```python
from build123d import *

# Parameters (mm, degrees)
BOSS_EXTRUDE1_DEPTH      = 25.5
BOSS_EXTRUDE1_DEPTH_BACK = 25.5
BOSS_EXTRUDE2_DEPTH      = 4
BOSS_EXTRUDE2_DEPTH_BACK = 4
SKETCH3_R                = 10
BOSS_EXTRUDE3_DEPTH      = 12.9
BOSS_EXTRUDE3_DEPTH_BACK = 12.9
SKETCH4_W                = 2.75
SKETCH4_H                = 8
SKETCH5_W                = 2.75
SKETCH5_H                = 8
SKETCH6_W                = 2.75
SKETCH6_H                = 8
SKETCH7_W                = 2.75
SKETCH7_H                = 8


with BuildPart() as part:
    # Sketch1 → Boss-Extrude1 (new body, two sides)
    with BuildSketch(Plane(origin=(0, 0, 0), x_dir=(0, 0, -1), z_dir=(1, 0, 0))) as boss_extrude1_sk:
        with BuildLine():
            Line((-15.5, 6.672), (-15.5, 0))
            Line((-15.5, 0), (15.5, 0))
            Line((15.5, 0), (15.5, 6.672))
            ThreePointArc((15.5, 6.672), (15.111037805, 7.611037805), (14.172, 8))
            Line((14.172, 8), (-14.172, 8))
            ThreePointArc((-14.172, 8), (-15.111037805, 7.611037805), (-15.5, 6.672))
        make_face()
    extrude(amount=BOSS_EXTRUDE1_DEPTH)
    extrude(boss_extrude1_sk.sketch, amount=-BOSS_EXTRUDE1_DEPTH_BACK)

    # Sketch2 → Boss-Extrude2 (add, two sides)
    with BuildSketch(Plane(origin=(0, 0, 0), x_dir=(0, 0, -1), z_dir=(1, 0, 0))) as boss_extrude2_sk:
        with BuildLine():
            Line((-21.283175656, 28.022230556), (-15.5, 6.656))
            ThreePointArc((-15.5, 6.656), (-15.106351514, 7.606351514), (-14.156, 8))
            Line((-14.156, 8), (14.675312578, 8))
            Line((14.675312578, 8), (-2.758705731, 36.074123248))
            ThreePointArc((-2.758705731, 36.074123248), (-2.824497754, 36.091976454), (-2.846947105, 36.027607565))
            ThreePointArc((-2.846947105, 36.027607565), (-8.013665194, 22.828896751), (-21.188967498, 28.055018845))
            ThreePointArc((-21.188967498, 28.055018845), (-21.251347415, 28.082515631), (-21.283175656, 28.022230556))
        make_face()
    extrude(amount=BOSS_EXTRUDE2_DEPTH)
    extrude(boss_extrude2_sk.sketch, amount=-BOSS_EXTRUDE2_DEPTH_BACK)

    # Sketch3 → Boss-Extrude3 (add, two sides)
    with BuildSketch(Plane(origin=(0, 0, 0), x_dir=(0, 0, -1), z_dir=(1, 0, 0))) as boss_extrude3_sk:
        with Locations((-12, 32)):
            Circle(SKETCH3_R)
    extrude(amount=BOSS_EXTRUDE3_DEPTH)
    extrude(boss_extrude3_sk.sketch, amount=-BOSS_EXTRUDE3_DEPTH_BACK)

    # Sketch4 → Cut-Revolve1 (revolve, cut)
    with BuildSketch(Plane.XY.offset(9)):
        with Locations((-20.375, 4)):
            Rectangle(SKETCH4_W, SKETCH4_H)
    revolve(axis=Axis((-19, 8, 9), (0, -1, 0)), mode=Mode.SUBTRACT)

    # Sketch5 → Cut-Revolve2 (revolve, cut)
    with BuildSketch(Plane.XY.offset(9)):
        with Locations((17.625, 4)):
            Rectangle(SKETCH5_W, SKETCH5_H)
    revolve(axis=Axis((19, 8, 9), (0, -1, 0)), mode=Mode.SUBTRACT)

    # Sketch6 → Cut-Revolve3 (revolve, cut)
    with BuildSketch(Plane.XY.offset(-9)):
        with Locations((-20.375, 4)):
            Rectangle(SKETCH6_W, SKETCH6_H)
    revolve(axis=Axis((-19, 8, -9), (0, -1, 0)), mode=Mode.SUBTRACT)

    # Sketch7 → Cut-Revolve4 (revolve, cut)
    with BuildSketch(Plane.XY.offset(-9)):
        with Locations((17.625, 4)):
            Rectangle(SKETCH7_W, SKETCH7_H)
    revolve(axis=Axis((19, 8, -9), (0, -1, 0)), mode=Mode.SUBTRACT)

    # Sketch8 → Cut-Revolve5 (revolve, cut)
    with BuildSketch(Plane.XY.offset(12)):
        Polygon((-12.9, 32), (-12.9, 39.22), (-12.611324865, 38.72), (12.611324865, 38.72), (12.9, 39.22), (12.9, 32), align=None)
    revolve(axis=Axis((12.9, 32, 12), (-1, 0, 0)), mode=Mode.SUBTRACT)

    # Sketch9 → Revolve1 (revolve)
    with BuildSketch(Plane.XY.offset(12)):
        Polygon((-12.9, 37.3), (-12.726794919, 37), (12.726794919, 37), (12.9, 37.3), (12.9, 38.7), (12.726794919, 39), (-12.726794919, 39), (-12.9, 38.7), align=None)
    revolve(axis=Axis((12.9, 32, 12), (-1, 0, 0)))


solid = part.part
```
CAD build for the part. Positions are in the model's coordinates, mm. A direction names the side the tool comes from. Round coordinates to 2 decimals unless told otherwise and drop trailing zeros. Loops run counter-clockwise (first coordinate to the right, second up) from the corner with the lowest first, then second, coordinate; pieces in that order, holes last. Notation, with made-up numbers: M 15,3.5 L 53,3.5 A16 ccw 53,14.5 Z; hole C 16,68 d6. An arc over 180 degrees is marked long. Use a Markdown table: item, result. Add a question column.
(1) Cut at D-D (x = 19). Give the cut face in (y, z), and give its area (3 significant figures).
(2) Cut at A-A (x = 6.5). Give the cut face in (y, z), and give its area (3 significant figures).
(3) Pull direction Z, two halves, no side cores. Call faces 6 (the face through (0, 3, -15.5)), 7 (the face through (-16.253, 4.056, 8.879)), 8 (the face through (15, 8, 0)): +Z half, -Z half, draft (parallel to the pull), parting line (faces both ways), or undercut.
(4) Drill centre lines: line 1 (Z direction, x = 19, y = 3); line 2 (X direction, y = 2.5, z = 9); line 3 (Y direction, x = 7.75, z = 12). Where is each one in solid material? Low to high.
(5) Cut at B-B (y = 3.5). Give the cut face in (x, z).
(6) Which spindle directions (+Z, -Z, +X, -X, +Y, -Y) get a long thin tool onto all of the face, cutting with end or side? Do faces 1 (the face through (-16.253, 4.056, -9.121)), 2 (the face through (-12.9, 32.5, 6.5)), 3 (the face through (-14.6, 7.62, 15.1)), 4 (the face through (14.9, 7.62, 15.1)), 5 (the face through (12.9, 25, 9)). Say none if no direction does.
(7) Cut at C-C (z = -9). Give the cut face in (x, y).
(8) Flat gauge pins, fed straight in: pin 1 (5.5 mm diameter, centred on x = -4.5, y = 3, fed in from +Z); pin 2 (16 mm diameter, centred on y = 32, z = 12, fed in from +X); pin 3 (11 mm diameter, centred on x = -19, z = -1, fed in from +Y). Where does each tip first touch, or does it go through?
Geometry says:
| question | item | result |
|---|---|---|
| 1 | outline | M 0,-15.5 L 6.67,-15.5 A1.33 ccw 8,-14.17 L 8,-11.75 L 0,-11.75 Z; M 0,-6.25 L 8,-6.25 L 8,6.25 L 0,6.25 Z; M 0,11.75 L 8,11.75 L 8,14.17 A1.33 ccw 6.67,15.5 L 0,15.5 Z |
| 1 | area | 159 mm² |
| 2 | outline | M 0,-15.5 L 6.67,-15.5 A1.33 ccw 8,-14.17 L 8,14.17 A1.33 ccw 6.67,15.5 L 0,15.5 Z; C 32,12 d20; hole C 32,12 d10 |
| 2 | area | 483 mm² |
| 3 | face 6 | -Z half |
| 3 | face 7 | undercut |
| 3 | face 8 | draft |
| 4 | line 1 | z = -15.5 to -11.75, -6.25 to 6.25, 11.75 to 15.5 |
| 4 | line 2 | x = -25.5 to -21.75, -16.25 to 16.25, 21.75 to 25.5 |
| 4 | line 3 | y = 0 to 8, 22 to 27, 37 to 42 |
| 5 | outline | M -25.5,-15.5 L 25.5,-15.5 L 25.5,15.5 L -25.5,15.5 Z; hole C -19,-9 d5.5; hole C -19,9 d5.5; hole C 19,-9 d5.5; hole C 19,9 d5.5 |
| 6 | face 1 | +Y, -Y |
| 6 | face 2 | +Z, -Z, -X, +Y |
| 6 | face 3 | +Z, -X |
| 6 | face 4 | +Z, +X |
| 6 | face 5 | +Z, -Z, +X, +Y |
| 7 | outline | M -25.5,0 L -21.75,0 L -21.75,8 L -25.5,8 Z; M -16.25,0 L 16.25,0 L 16.25,8 L 4,8 L 4,17.14 L -4,17.14 L -4,8 L -16.25,8 Z; M 21.75,0 L 25.5,0 L 25.5,8 L 21.75,8 Z |
| 8 | pin 1 | stops at z = 15.5 |
| 8 | pin 2 | stops at x = 12.9 |
| 8 | pin 3 | stops at y = 8 |
